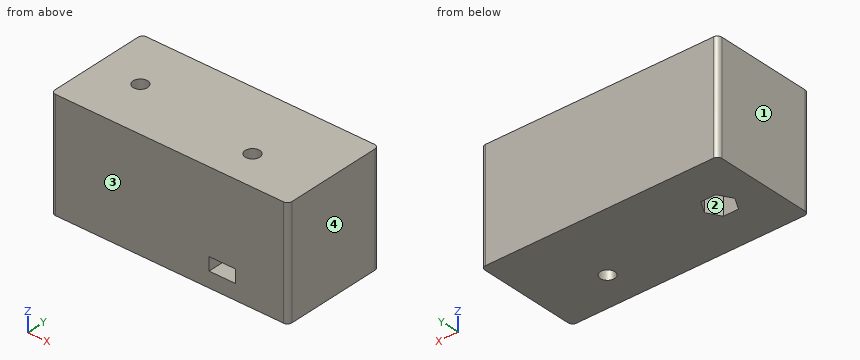
Solid Edge part; units mm, degrees
sketch "Sketch1" plane through (0, 0, 0) normal (0, 0, 1) x (1, 0, 0)
  line L0 (-27, -12) -> (27, -12)
  line L1 (27, -12) -> (27, 12)
  line L2 (27, 12) -> (-27, 12)
  line L3 (-27, 12) -> (-27, -12)
  dimension "D1" = 27
  dimension "D2" = 27
extrude "Ajout_matière_1" add sketch "Sketch1" along normal mid plane 25
fillet "Congé_1" radius 1 4 edges at (27, -12, 0) (27, 12, 0) (-27, -12, 0) (-27, 12, 0)
hole "Perçage_5" at (12, -4, 12.5) direction (0, 0, -1) diameter 3.3 end up to next
sketch "Sketch2" plane through (0, -12, 0) normal (0, -1, 0) x (0, 0, -1)
  line L0 (6, 9) -> (9, 9)
  line L1 (9, 9) -> (9, 15)
  line L2 (9, 15) -> (6, 15)
  line L3 (6, 15) -> (6, 9)
  dimension "D1" = 9
  dimension "D2" = 9
  dimension "D3" = 9
extrude "Enlèvement_matière_3" cut sketch "Sketch2" against normal blind 11.5
sketch "Sketch3" plane through (0, 0, -12.5) normal (0, 0, -1) x (0, 1, 0)
  line L0 (3, -15.2679) -> (0, -13.5359)
  line L1 (0, -13.5359) -> (-3, -15.2679)
  line L2 (-3, -15.2679) -> (-3, -18.7321)
  line L3 (-3, -18.7321) -> (0, -20.4641)
  line L4 (0, -20.4641) -> (3, -18.7321)
  line L5 (3, -18.7321) -> (3, -15.2679)
  dimension "D1" = 3
extrude "Enlèvement_matière_5" cut sketch "Sketch3" against normal blind 15
hole "Perçage_6" at (-17, 0, 2.5) direction (0, 0, 1) diameter 3.3 end up to next
properties material "Plastique ABS, haute performance"
Part model, mm, in its own coordinate system. Face numbers are marked on the shaded views. Round coordinates to 2 decimals unless told otherwise and drop trailing zeros. Write each loop counter-clockwise with the first axis right and the second up, starting at its lowest first coordinate (ties: lowest second). Pieces come first, ordered by that corner, then holes. Notation, with made-up numbers: (10.25, 9.25) - (45.25, 9.25) arc R32 ccw to (45.25, 40.25) - close; hole circle Ø6 at (63.5, -3). An arc over 180 degrees is marked (long way). Use CSV: the item, a comma, the result in double quotes.
Item 1: Slice it at B-B, the plane z = -11. Write the cut outline in (x, y), then the cut area to 3 significant figures.
Results list:
outline,"(-27, -11) arc R1 ccw to (-26, -12) - (26, -12) arc R1 ccw to (27, -11) - (27, 11) arc R1 ccw to (26, 12) - (-26, 12) arc R1 ccw to (-27, 11) - close; hole (-20.46, 0) - (-18.73, -3) - (-15.27, -3) - (-13.54, 0) - (-15.27, 3) - (-18.73, 3) - close; hole circle Ø3.3 at (12, -4)"
area,"1,260 mm²"
Item 2: Wall check: L1, parallel to X at y = -4, z = 0.5; L2, parallel to X at y = 0, z = 7.75; L3, parallel to Y at x = -16, z = -7. Give the ranges that are in metal, low to high.
Results list:
L1,"x = -27 to 10.35, 13.65 to 27"
L2,"x = -27 to -18.65, -15.35 to 27"
L3,"y = -12 to -3, 3 to 12"
Item 3: Slice it at C-C, the plane x = 12. Write the cut outline in (y, z), then the cut area to 3 significant figures.
Results list:
outline,"(-12, -12.5) - (-5.65, -12.5) - (-5.65, -9) - (-12, -9) - close; (-12, -6) - (-5.65, -6) - (-5.65, 12.5) - (-12, 12.5) - close; (-2.35, -12.5) - (12, -12.5) - (12, 12.5) - (-2.35, 12.5) - (-2.35, -6) - (-0.5, -6) - (-0.5, -9) - (-2.35, -9) - close"
area,"493 mm²"
Item 4: Slice it at A-A, the plane x = -17. Write the cut outline in (y, z), then the cut area to 3 significant figures.
Results list:
outline,"(-12, -12.5) - (-3, -12.5) - (-3, 2.5) - (-1.65, 2.5) - (-1.65, 12.5) - (-12, 12.5) - close; (1.65, 2.5) - (3, 2.5) - (3, -12.5) - (12, -12.5) - (12, 12.5) - (1.65, 12.5) - close"
area,"477 mm²"
Item 5: Flat gauge pin, fed straight in: P1, Ø1.8, axis at x = -16.5, y = -1, coming from the -Z side. Where does the tip first touch, or does it go through?
Results list:
P1,"stops at z = 2.5"
Item 6: Pull direction X, two halves, no side cores. Call the marked faces 1, 2, 3 and 4: pulls with the +X half, pulls with the -X half, needs draft (parallel to the pull), parting line crosses it, or undercut.
Results list:
face 1,"pulls with the -X half"
face 2,"undercut"
face 3,"needs draft"
face 4,"pulls with the +X half"
